Geometry check sheet. Reference: the model listing, model coordinates, mm. Coordinates: 2 decimals unless noted, no trailing zeros. Loops run counter-clockwise (first coordinate to the right, second up) from the corner with the lowest first, then second, coordinate; pieces in that order, holes last.
from build123d import *

# Parameters (mm, degrees)
F1_DEPTH = 4.953
F2_R     = 3.429
F3_DEPTH = 25.4


with BuildPart() as f1:
    # F0 (on Front) → F1 (new body)
    with BuildSketch(Plane.XZ):
        with BuildLine():
            Line((-12.5887309267, 0), (12.8112690733, 0))
            Line((12.8112690733, 0), (12.8112690733, 63.5))
            ThreePointArc((12.8112690733, 63.5), (0.1112690733, 50.8), (-12.5887309267, 63.5))
            Line((-12.5887309267, 63.5), (-12.5887309267, 0))
        make_face()
        with BuildLine():
            ThreePointArc((-12.5887309267, 63.5), (0.1112690733, 50.8), (12.8112690733, 63.5))
            Line((12.8112690733, 63.5), (-12.5887309267, 63.5))
        make_face()
        with BuildLine():
            Line((-12.5887309267, 63.5), (12.8112690733, 63.5))
            ThreePointArc((12.8112690733, 63.5), (0.1112690733, 76.2), (-12.5887309267, 63.5))
        make_face()
    extrude(amount=F1_DEPTH)

    # F2 (on face) → F3 (cut)
    with BuildSketch(Plane.XZ.offset(4.953)):
        with Locations((0, 12.7)):
            Circle(F2_R)
        with Locations((0, 38.1)):
            Circle(F2_R)
        with Locations((0, 63.5)):
            Circle(F2_R)
    extrude(amount=-F3_DEPTH, mode=Mode.SUBTRACT)


solid = f1.part
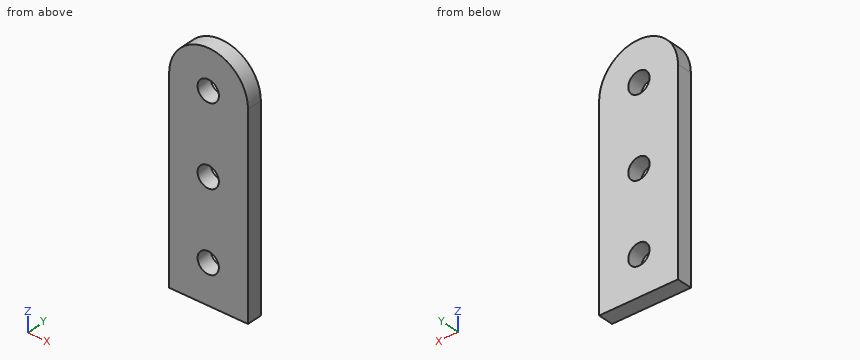
1) Depth check by flat-ended pin: pin 1 (1.5 mm diameter, centred on y = -4, z = 66, fed in from -X); pin 2 (1.5 mm diameter, centred on x = 8, y = -4, fed in from +Z); pin 3 (11 mm diameter, centred on x = 0, z = 38.1, fed in from +Y). Enter the tip coordinate at first touch or a pass-through.
Data:
pin 1: stops at x = -12.47
pin 2: stops at z = 74
pin 3: stops at y = 0
2) Section check D-D on z = 71. Record the cut outline in (x, y).
Data:
outline: (-10.14, -4.95) - (10.36, -4.95) - (10.36, 0) - (-10.14, 0) - close
3) Section check A-A on y = -0.8. Record the cut outline in (x, z).
Data:
outline: (-12.59, 0) - (12.81, 0) - (12.81, 63.5) arc R12.7 ccw to (-12.59, 63.5) - close; hole circle Ø6.86 at (0, 12.7); hole circle Ø6.86 at (0, 38.1); hole circle Ø6.86 at (0, 63.5)
4) Section check C-C on x = 0. Record the cut outline in (y, z), and give its area (3 significant figures).
Data:
outline: (-4.95, 0) - (0, 0) - (0, 9.27) - (-4.95, 9.27) - close; (-4.95, 16.13) - (0, 16.13) - (0, 34.67) - (-4.95, 34.67) - close; (-4.95, 41.53) - (0, 41.53) - (0, 60.07) - (-4.95, 60.07) - close; (-4.95, 66.93) - (0, 66.93) - (0, 76.2) - (-4.95, 76.2) - close
area: 276 mm2
5) Material ranges on probe 1 along Z at (x, y) = (0, -1.5); probe 2 along Z at (x, y) = (-3, -3.65); probe 3 along X at (y, z) = (-3, 38.5), recorded low to high.
Data:
probe 1: z = 0 to 9.27, 16.13 to 34.67, 41.53 to 60.07, 66.93 to 76.2
probe 2: z = 0 to 11.04, 14.36 to 36.44, 39.76 to 61.84, 65.16 to 75.81
probe 3: x = -12.59 to -3.41, 3.41 to 12.81
6) Section check B-B on z = 12.7. Record the cut outline in (x, y).
Data:
outline: (-12.59, -4.95) - (-3.43, -4.95) - (-3.43, 0) - (-12.59, 0) - close; (3.43, -4.95) - (12.81, -4.95) - (12.81, 0) - (3.43, 0) - close
